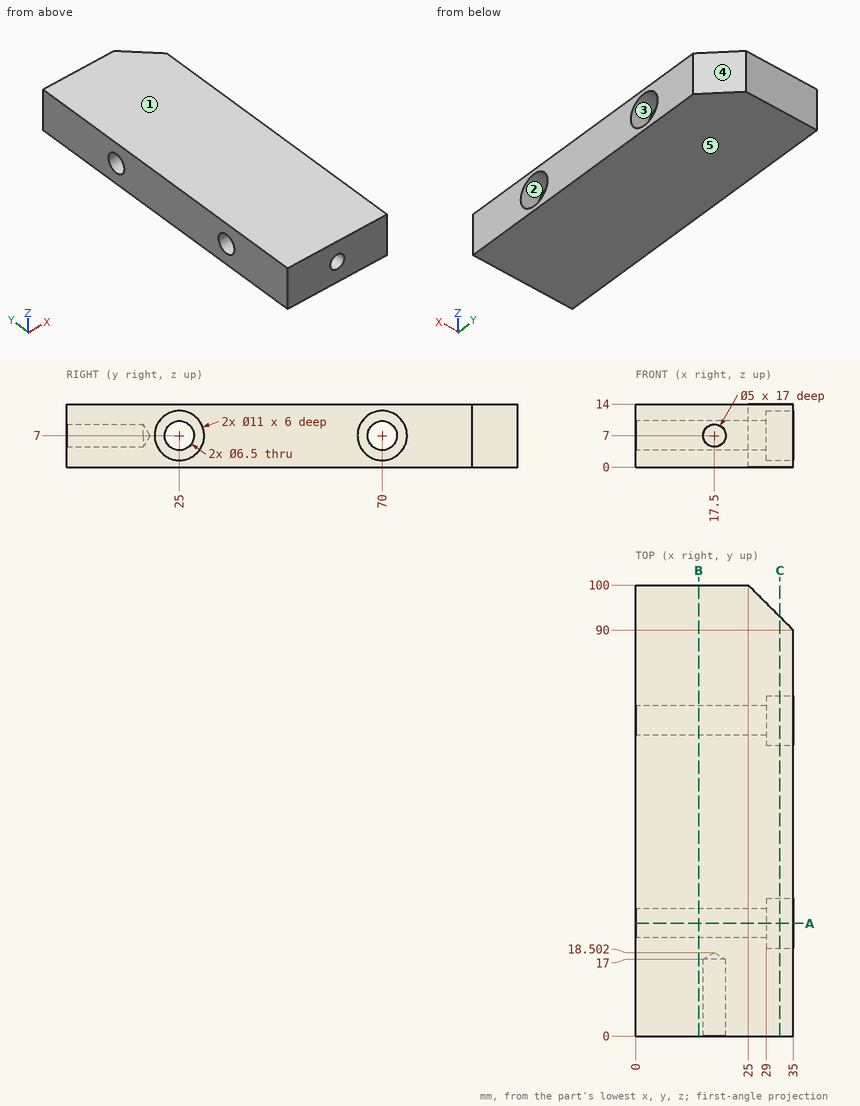
Input: dimensioned drawing with shaded views. Units: mm. Origin: part minimum x, y, z. A direction names the side the tool comes from. Coordinates: 2 decimals unless noted, no trailing zeros. Order: outer loops, then holes, each group sorted by start corner. A loop starts at its lowest first (then second) coordinate and runs counter-clockwise, first axis right, second up.
1. Draft query along Y for the marked faces 3, 4 and 5. Return one class per face: +Y half, -Y half, draft (parallel to the pull), parting line (faces both ways), or undercut.
Checked values:
face 3: undercut
face 4: +Y half
face 5: draft
2. Cut plane B-B, the plane x = 14. Return loops of the section in (y, z), plus the area to 3 significant figures.
Checked values:
outline: (0, 0) - (100, 0) - (100, 14) - (0, 14) - close; hole circle Ø6.5 at (25, 7); hole circle Ø6.5 at (70, 7)
area: 1,330 mm2
3. Contact query for a flat-ended pin moving along its axis: P1, Ø3.5, axis at y = 72.5, z = 9.5, coming from the +X side. Output: stop coordinate, or through.
Checked values:
P1: stops at x = 29
4. Cut plane C-C, the plane x = 32. Return loops of the section in (y, z).
Checked values:
outline: (0, 0) - (93, 0) - (93, 14) - (0, 14) - close; hole circle Ø11 at (25, 7); hole circle Ø11 at (70, 7)
5. Ray query, line 1 along Y through (x, z) = (14, 7); line 2 along Y through (x, z) = (10.5, 9); line 3 along Z through (x, y) = (17.5, 9.25). Return the intervals inside material, ascending.
Checked values:
line 1: y = 0 to 21.75, 28.25 to 66.75, 73.25 to 100
line 2: y = 0 to 22.44, 27.56 to 67.44, 72.56 to 100
line 3: z = 0 to 4.5, 9.5 to 14
6. Cut plane A-A, the plane y = 25. Return loops of the section in (x, z).
Checked values:
outline: (0, 0) - (35, 0) - (35, 1.5) - (29, 1.5) - (29, 3.75) - (0, 3.75) - close; (0, 10.25) - (29, 10.25) - (29, 12.5) - (35, 12.5) - (35, 14) - (0, 14) - close
7. Access query for the marked faces 1 and 2. Directions: +Z, -Z, +X, -X, +Y, -Y. A direction counts if a zero-diameter tool reaches every point of the face in a straight line with its end or side. Return the directions, or none.
Checked values:
face 1: +Z, +X, -X, +Y, -Y
face 2: +X
